Geometry check sheet. Reference: drawing and pictorial views, mm from the part's lowest x, y, z. Give positions to 0.01 mm unless a question says otherwise; leave off trailing zeros. Write each loop counter-clockwise with the first axis right and the second up, starting at its lowest first coordinate (ties: lowest second). Pieces come first, ordered by that corner, then holes. Notation, with made-up numbers: (19, 11) -> (42, 11) arc R9 ccw to (42, 24) -> close; hole circle Ø9 at (36, 53.25). An arc over 180 degrees is marked (long way). Return JSON: item names as keys, results as strings.
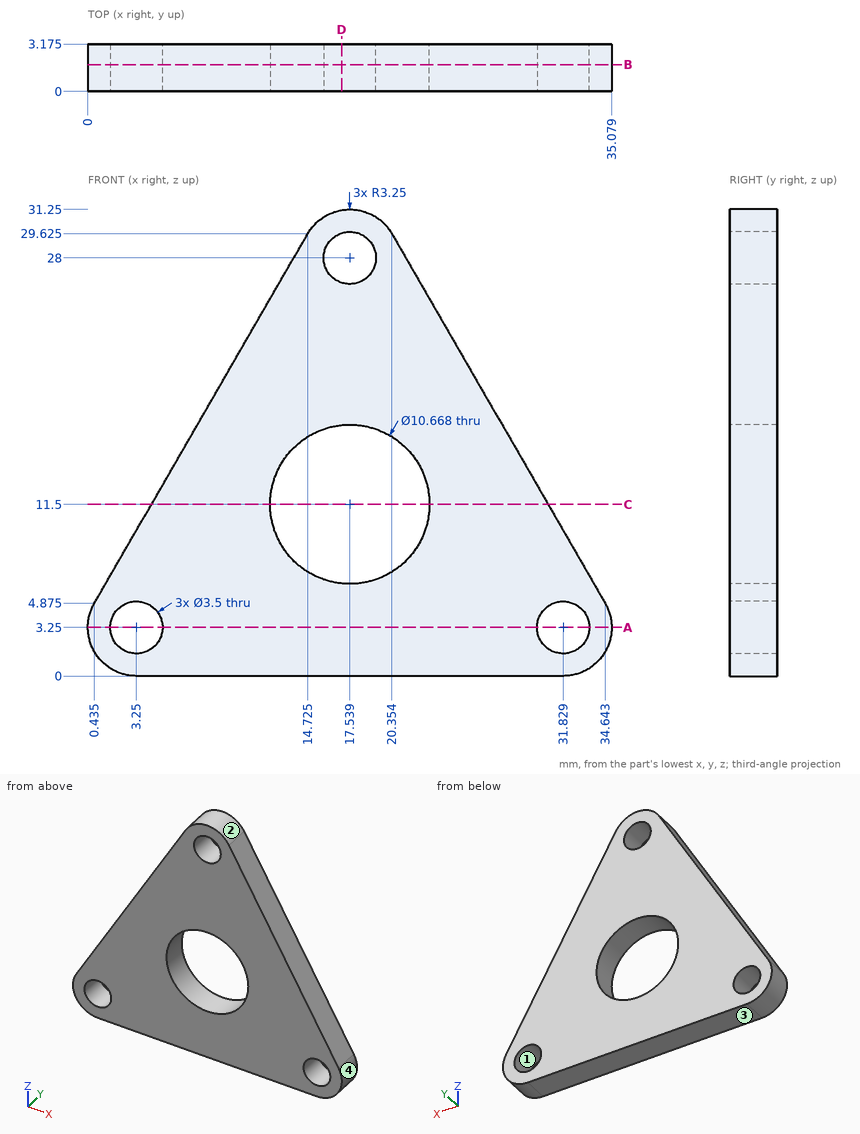
(1) Cross-section at C-C on z = 11.5. Enter the section's corners in (x, y) (1 decimal).
Reply:
{"outline": "(4.3, 0) -> (12.2, 0) -> (12.2, 3.2) -> (4.3, 3.2) -> close; (22.9, 0) -> (30.8, 0) -> (30.8, 3.2) -> (22.9, 3.2) -> close"}
(2) Cross-section at B-B on y = 1.8. State how many separate pieces and enclosed holes the cut face has, then the cut area to 3 significant figures.
Reply:
{"separate pieces": "1", "enclosed holes": "4", "area": "547 mm^2"}
(3) Thickness scan on L1, parallel to X at y = 1.5, z = 3.25; L2, parallel to X at y = 0.9, z = 7.5; L3, parallel to X at y = 1.85, z = 29 (1 decimal). Record the ranges inside material, lowest first.
Reply:
{"L1": "0 to 1.5, 5 to 30.08, 33.58 to 35.08", "L2": "1.95 to 14.01, 21.07 to 33.13", "L3": "14.4 to 16.1, 19 to 20.7"}
(4) Cross-section at A-A on z = 3.25. Enter the section's corners in (x, y) (1 decimal).
Reply:
{"outline": "(0, 0) -> (1.5, 0) -> (1.5, 3.2) -> (0, 3.2) -> close; (5, 0) -> (30.1, 0) -> (30.1, 3.2) -> (5, 3.2) -> close; (33.6, 0) -> (35.1, 0) -> (35.1, 3.2) -> (33.6, 3.2) -> close"}
(5) Cross-section at D-D on x = 17. Enter the section's corners in (y, z) (1 decimal).
Reply:
{"outline": "(0, 0) -> (3.2, 0) -> (3.2, 6.2) -> (0, 6.2) -> close; (0, 16.8) -> (3.2, 16.8) -> (3.2, 26.3) -> (0, 26.3) -> close; (0, 29.7) -> (3.2, 29.7) -> (3.2, 31.2) -> (0, 31.2) -> close"}
(6) Release check for a two-part mould opening along X. For the marked faces 1, 2, 3 and 4 record: pulls with the +X half, pulls with the -X half, needs draft (parallel to the pull), parting line crosses it, or undercut.
Reply:
{"face 1": "undercut", "face 2": "parting line crosses it", "face 3": "needs draft", "face 4": "pulls with the +X half"}
